from build123d import *

# Parameters (mm, degrees)
SKETCH1_W           = 60
SKETCH1_H           = 90
BOSS_EXTRUDE1_DEPTH = 15
SKETCH2_R           = 30
SKETCH2_R_2         = 15
BOSS_EXTRUDE2_DEPTH = 30
CUT_EXTRUDE1_START  = -30
CUT_EXTRUDE1_DEPTH  = 30
SKETCH4_R           = 8
BOSS_EXTRUDE4_DEPTH = 15
BOSS_EXTRUDE5_START = -15
SKETCH8_R           = 8
BOSS_EXTRUDE5_DEPTH = 15


with BuildPart() as part:
    # Sketch1 → Boss-Extrude1 (new body)
    with BuildSketch(Plane.XY):
        Rectangle(SKETCH1_W, SKETCH1_H)
    extrude(amount=BOSS_EXTRUDE1_DEPTH)

    # Sketch2 → Boss-Extrude2 (add)
    with BuildSketch(Plane.XY.offset(15)):
        Circle(SKETCH2_R)
        Circle(SKETCH2_R_2, mode=Mode.SUBTRACT)
    extrude(amount=BOSS_EXTRUDE2_DEPTH)

    # Sketch3 → Cut-Extrude1 (cut)
    with BuildSketch(Plane.XY.offset(45).offset(CUT_EXTRUDE1_START)):
        with BuildLine():
            Line((-4, -18), (4, -18))
            Line((4, -18), (4, -14.456832295))
            ThreePointArc((4, -14.456832295), (0, 15), (-4, -14.456832295))
            Line((-4, -14.456832295), (-4, -18))
        make_face()
    extrude(amount=CUT_EXTRUDE1_DEPTH, mode=Mode.SUBTRACT)

    # Sketch4 → Boss-Extrude4 (add)
    with BuildSketch(Plane(origin=(0, 45, 0), x_dir=(1, 0, 0), z_dir=(0, 1, 0))):
        with BuildLine():
            Line((-30, 0), (-22.79450882, 38.067632254))
            ThreePointArc((-22.79450882, 38.067632254), (0, 58), (22.79450882, 38.067632254))
            Line((22.79450882, 38.067632254), (30, 0))
            Line((30, 0), (-30, 0))
        make_face()
        with Locations(Location((0, 35, 0), (0, 0, 270))):
            Circle(SKETCH4_R, mode=Mode.SUBTRACT)
    extrude(amount=-BOSS_EXTRUDE4_DEPTH)

    # Sketch8 → Boss-Extrude5 (add)
    with BuildSketch(Plane.XZ.offset(45).offset(BOSS_EXTRUDE5_START)):
        with BuildLine():
            Line((30, 0), (-30, 0))
            Line((-30, 0), (-22.800687568, -38.021364997))
            Line((-22.800687568, -38.021364997), (-22.326909292, -40.523506265))
            ThreePointArc((-22.326909292, -40.523506265), (0, -58), (22.326909292, -40.523506265))
            Line((22.326909292, -40.523506265), (22.800687568, -38.021364997))
            Line((22.800687568, -38.021364997), (30, 0))
        make_face()
        with Locations(Location((0, -35, 0), (0, 0, 90))):
            Circle(SKETCH8_R, mode=Mode.SUBTRACT)
    extrude(amount=BOSS_EXTRUDE5_DEPTH)


solid = part.part
The listing builds one solid part. Answer for the finished solid, in the listing's coordinates (mm). A direction names the side the tool comes from. Give positions to 0.01 mm unless a question says otherwise; leave off trailing zeros. Write each loop counter-clockwise with the first axis right and the second up, starting at its lowest first coordinate (ties: lowest second). Pieces come first, ordered by that corner, then holes.
Item 1: Section D-D, the plane z = 28 is taken. Write down the section's boundary in (x, y), plus the area to 3 significant figures.
Item 2: Which of the six approach directions +Z, -Z, +X, -X, +Y, -Y give full straight-line access (tool end or side, diameter ignored) to faces 1 (the cylindrical face through (-29.97, 1.32, 29.79)), 2 (the flat face through (0, 0, 0)), 3 (the flat face through (0, 33, 15))?
Item 3: Section B-B, the plane z = -11 is taken. Write down the section's boundary in (x, y).
Item 4: Flat-ended cylindrical pins translate along their axes: P1, Ø15, axis at x = -3, y = 2.5, coming from the +Z side; P2, Ø2, axis at y = 4.5, z = 19, coming from the -X side; P3, Ø1, axis at y = -22.5, z = 24, coming from the -X side; P4, Ø9.5, axis at x = 0, z = -35, coming from the +Y side. Find the tip coordinate at first contact, or state that the pin passes through.
Item 5: Determine the mould class of faces 4 (the cylindrical face through (4.868, -37.395, -41.349)), 5 (the flat face through (0, -32, 15)), 6 (the flat face through (0, -18, 30)) for opening direction Z: released by +Z, released by -Z, zero draft, split by the parting line, or undercut.
Item 6: Section A-A, the plane x = 0 is taken. Write down the section's boundary in (y, z).
Item 7: Section C-C, the plane y = -35 is taken. Write down the section's boundary in (x, z).
Item 8: Find the intervals of material crossed by line 1 along Y through (x, z) = (-14.5, -29); line 2 along Y through (x, z) = (0, 28.5); line 3 along Z through (x, y) = (2.5, 2.5), in increasing order.
Completed:
1. outline: circle Ø60 at (0, 0); hole (-4, -18) - (4, -18) - (4, -14.46) arc R15 ccw (long way) to (-4, -14.46) - close
1. area: 2,100 mm2
2. face 1: +Z
2. face 2: -Z, +X, -X
2. face 3: +Z, +Y
3. outline: (-27.92, -45) - (27.92, -45) - (27.92, -30) - (-27.92, -30) - close; (-27.92, 30) - (27.92, 30) - (27.92, 45) - (-27.92, 45) - close
4. P1: stops at z = 15
4. P2: stops at x = -29.8
4. P3: stops at x = -20.4
4. P4: passes through
5. face 4: undercut
5. face 5: released by +Z
5. face 6: zero draft
6. outline: (-45, -58) - (-30, -58) - (-30, -43) - (-45, -43) - close; (-45, -27) - (-30, -27) - (-30, 0) - (30, 0) - (30, -27) - (45, -27) - (45, 15) - (30, 15) - (30, 45) - (15, 45) - (15, 15) - (-18, 15) - (-18, 45) - (-30, 45) - (-30, 15) - (-45, 15) - close; (30, -58) - (45, -58) - (45, -43) - (30, -43) - close
7. outline: (-30, 0) - (-22.33, -40.52) arc R23 ccw to (22.33, -40.52) - (30, 0) - (30, 15) - (-30, 15) - close; hole circle Ø16 at (0, -35)
8. line 1: y = -45 to -30, 30 to 45
8. line 2: y = -30 to -18, 15 to 30
8. line 3: z = 0 to 15
